```python
from build123d import *

# Parameters (mm, degrees)
F1_DEPTH = 3


with BuildPart() as f1:
    # F0 (on Top) → F1 (new body)
    with BuildSketch(Plane.XY):
        Polygon((25, 10), (-25, 10), (-25, 7), (-23, 7), (-23, 2), (-25, 2), (-25, 0), (-25, -2), (-23, -2), (-23, -7), (-25, -7), (-25, -10), (25, -10), (25, -7), (23, -7), (23, -2), (25, -2), (25, 0), (25, 2), (23, 2), (23, 7), (25, 7), align=None)
    extrude(amount=F1_DEPTH)


solid = f1.part
```
Verification items for the finished model (mm, model axes). A direction names the side the tool comes from. Round coordinates to 2 decimals unless told otherwise and drop trailing zeros. Loops run counter-clockwise (first coordinate to the right, second up) from the corner with the lowest first, then second, coordinate; pieces in that order, holes last. Notation, with made-up numbers: (29.25, 50.25) -> (82.25, 50.25) arc R17 ccw to (82.25, 56.25) -> close; hole circle Ø7 at (-26, 16.25). An arc over 180 degrees is marked (long way). Answer as a JSON object with one key per item and string values.
Q1. Access from +Z, -Z, +X, -X, +Y, -Y to the whole of each face (thin tool, end or side, straight path). Record for faces 1 (the flat face through (24, 7, 1)), 2 (the flat face through (-23, 5, 1)), 3 (the flat face through (25, 0, 1)).
Data:
{"face 1": "+Z, -Z, +X", "face 2": "+Z, -Z, -X", "face 3": "+Z, -Z, +X, +Y, -Y"}
Q2. Scan line: line 1 (X direction, y = 6.5, z = 1.85). Record every from-to range of solid material in increasing order. Write a range as from..to.
Data:
{"line 1": "x = -23..23"}
Q3. Section check A-A (z = 2.15). Record the boundary of the cut face in (x, y), then the cut area to 3 significant figures.
Data:
{"outline": "(-25, -10) -> (25, -10) -> (25, -7) -> (23, -7) -> (23, -2) -> (25, -2) -> (25, 2) -> (23, 2) -> (23, 7) -> (25, 7) -> (25, 10) -> (-25, 10) -> (-25, 7) -> (-23, 7) -> (-23, 2) -> (-25, 2) -> (-25, -2) -> (-23, -2) -> (-23, -7) -> (-25, -7) -> close", "area": "960 mm2"}
Q4. Section check B-B (y = -6.5). Record the boundary of the cut face in (x, z).
Data:
{"outline": "(-23, 0) -> (23, 0) -> (23, 3) -> (-23, 3) -> close"}
Q5. Draft check along Y on faces 4 (the flat face through (-23, -4, 1)), 5 (the flat face through (0, -10, 1)), 6 (the flat face through (0, 10, 1)). Enter one of: pulls with the +Y half, pulls with the -Y half, needs draft (parallel to the pull), parting line crosses it, or undercut.
Data:
{"face 4": "undercut", "face 5": "pulls with the -Y half", "face 6": "pulls with the +Y half"}
Q6. Go/stop test with flat-tipped pins: P1, Ø0.9, axis at y = -4, z = 2, coming from the +X side; P2, Ø1.5, axis at y = -4.5, z = 1, coming from the -X side. Record where each tip stops, or that it passes through.
Data:
{"P1": "stops at x = 23", "P2": "stops at x = -23"}
